CAD build for the part. Positions are in the model's coordinates, mm. Face numbers are marked on the shaded views. A direction names the side the tool comes from. Coordinates: 2 decimals unless noted, no trailing zeros. Order: outer loops, then holes, each group sorted by start corner. A loop starts at its lowest first (then second) coordinate and runs counter-clockwise, first axis right, second up. Notation, with made-up numbers: M -11.5,12.5 L 25.5,12.5 A21 ccw 25.5,23.5 Z; hole C -34,36.25 d6. An arc over 180 degrees is marked long. Write item = value, one per line.
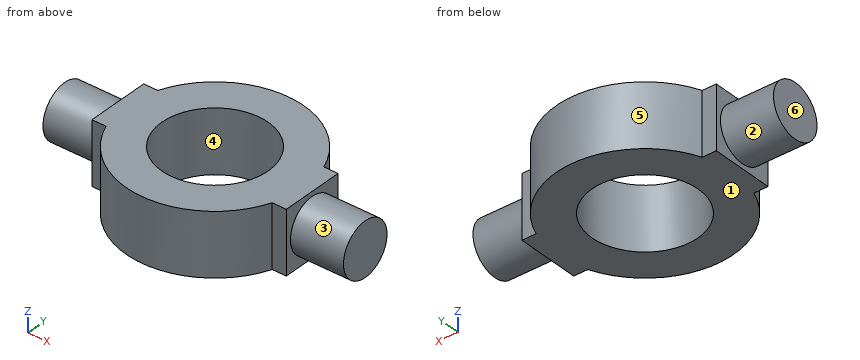
from build123d import *

# Parameters (mm, degrees)
F1_DEPTH = 17.75
F3_R     = 15.1
F4_DEPTH = 30
F6_R     = 15.1
F7_DEPTH = 30
F10_D    = 60.1


with BuildPart() as f1:
    # F0 (on Top) → F1 (new body, symmetric)
    with BuildSketch(Plane.XY):
        with BuildLine():
            ThreePointArc((46.9881634031, -17.95), (49.4651120446, -9.1264829157), (50.3, 0))
            ThreePointArc((50.3, 0), (49.4651120446, 9.1264829157), (46.9881634031, 17.95))
            Line((46.9881634031, 17.95), (-46.9881634031, 17.95))
            ThreePointArc((-46.9881634031, 17.95), (-50.3, 0), (-46.9881634031, -17.95))
            Line((-46.9881634031, -17.95), (46.9881634031, -17.95))
        make_face()
        with BuildLine():
            Line((-46.9881634031, 17.95), (46.9881634031, 17.95))
            ThreePointArc((46.9881634031, 17.95), (0, 50.3), (-46.9881634031, 17.95))
        make_face()
        with BuildLine():
            ThreePointArc((46.9881634031, 17.95), (49.4651120446, 9.1264829157), (50.3, 0))
            ThreePointArc((50.3, 0), (49.4651120446, -9.1264829157), (46.9881634031, -17.95))
            Line((46.9881634031, -17.95), (55, -17.95))
            Line((55, -17.95), (55, 17.95))
            Line((55, 17.95), (46.9881634031, 17.95))
        make_face()
        with BuildLine():
            ThreePointArc((-46.9881634031, -17.95), (0, -50.3), (46.9881634031, -17.95))
            Line((46.9881634031, -17.95), (-46.9881634031, -17.95))
        make_face()
        with BuildLine():
            ThreePointArc((-46.9881634031, -17.95), (-50.3, 0), (-46.9881634031, 17.95))
            Line((-46.9881634031, 17.95), (-55, 17.95))
            Line((-55, 17.95), (-55, -17.95))
            Line((-55, -17.95), (-46.9881634031, -17.95))
        make_face()
    extrude(amount=F1_DEPTH, both=True)

    # F3 (on offset) → F4 (join)
    with BuildSketch(Plane.YZ.offset(55)):
        Circle(F3_R)
    extrude(amount=F4_DEPTH)

    # F6 (on offset) → F7 (join)
    with BuildSketch(Plane(origin=(-55, 0, 0), x_dir=(0, -1, 0), z_dir=(-1, 0, 0))):
        Circle(F6_R)
    extrude(amount=F7_DEPTH)

    # F10 (through all)
    with Locations(Plane(origin=(0, 0, -17.75), x_dir=(1, 0, 0), z_dir=(0, 0, -1))):
        with Locations((0, 0)):
            Hole(F10_D / 2)


solid = f1.part
(1) Wall check: line 1 (Y direction, x = 0, z = -5.5); line 2 (X direction, y = -14, z = 10.5); line 3 (Y direction, x = 11, z = 13). Give the ranges that are in metal, low to high. Write a range as from..to.
Evaluation:
line_1 = -50.3..-30.05, 30.05..50.3
line_2 = -55..-26.59, 26.59..55
line_3 = -49.08..-27.96, 27.96..49.08
(2) Slice it at C-C, the plane z = 0. Write the cut outline in (x, y).
Evaluation:
outline = M -85,-15.1 L -55,-15.1 L -55,-17.95 L -46.99,-17.95 A50.3 ccw 46.99,-17.95 L 55,-17.95 L 55,-15.1 L 85,-15.1 L 85,15.1 L 55,15.1 L 55,17.95 L 46.99,17.95 A50.3 ccw -46.99,17.95 L -55,17.95 L -55,15.1 L -85,15.1 Z; hole C 0,0 d60.1
(3) Pin check, flat tips, straight feed: pin 1 Ø8 at (x, z) = (-12.5, -1.5) entering from -Y; pin 2 Ø4 at (x, z) = (52.5, -4) entering from -Y; pin 3 Ø1.5 at (x, y) = (-57.5, 10.5) entering from -Z. Stop position of each tip, or through.
Evaluation:
pin_1 = -49.58
pin_2 = -17.95
pin_3 = -11.53
(4) Tool access for the marked faces 1, 2 and 3: list every direction of +Z, -Z, +X, -X, +Y, -Y with a clear straight run to the whole face (end or side of a thin tool).
Evaluation:
face_1 = -Z, +X, -X, +Y, -Y
face_2 = -X
face_3 = +X
(5) Slice it at D-D, the plane y = 24.5. Write the cut outline in (x, z).
Evaluation:
outline = M -43.93,-17.75 L -17.4,-17.75 L -17.4,17.75 L -43.93,17.75 Z; M 17.4,-17.75 L 43.93,-17.75 L 43.93,17.75 L 17.4,17.75 Z
(6) Slice it at B-B, the plane y = 0. Write the cut outline in (x, z).
Evaluation:
outline = M -85,-15.1 L -55,-15.1 L -55,-17.75 L -30.05,-17.75 L -30.05,17.75 L -55,17.75 L -55,15.1 L -85,15.1 Z; M 30.05,-17.75 L 55,-17.75 L 55,-15.1 L 85,-15.1 L 85,15.1 L 55,15.1 L 55,17.75 L 30.05,17.75 Z
(7) Pull direction Y, two halves, no side cores. Call the marked faces 4, 5 and 6: +Y half, -Y half, draft (parallel to the pull), parting line (faces both ways), or undercut.
Evaluation:
face_4 = undercut
face_5 = +Y half
face_6 = draft
(8) Slice it at A-A, the plane x = 0. Write the cut outline in (y, z), then the cut area to 3 significant figures.
Evaluation:
outline = M -50.3,-17.75 L -30.05,-17.75 L -30.05,17.75 L -50.3,17.75 Z; M 30.05,-17.75 L 50.3,-17.75 L 50.3,17.75 L 30.05,17.75 Z
area = 1,440 mm²
